```python
from build123d import *

# Parameters (mm, degrees)
SKETCH007_W     = 116.5
SKETCH007_H     = 84
PAD002_DEPTH    = 2
SKETCH008_W     = 112.5
SKETCH008_H     = 80
PAD003_DEPTH    = 2
SKETCH009_W     = 108.5
SKETCH009_H     = 76
POCKET004_DEPTH = 2
FILLET008_R     = 1
FILLET009_R     = 1


with BuildPart() as part:
    # Sketch007 → Pad002 (new body)
    with BuildSketch(Plane(origin=(0, 0, 0), x_dir=(1, 0, 0), z_dir=(0, 0, -1))):
        with Locations((58.25, 42)):
            Rectangle(SKETCH007_W, SKETCH007_H)
    extrude(amount=PAD002_DEPTH)

    # Sketch008 (on Face5 of Pad002) → Pad003 (new body)
    with BuildSketch(Plane.XY):
        with Locations((58.25, -42)):
            Rectangle(SKETCH008_W, SKETCH008_H)
    extrude(amount=PAD003_DEPTH)

    # Sketch009 (on Face11 of Pad003) → Pocket004 (cut)
    with BuildSketch(Plane.XY.offset(2)):
        with Locations((58.25, -42)):
            Rectangle(SKETCH009_W, SKETCH009_H)
    extrude(amount=-POCKET004_DEPTH, mode=Mode.SUBTRACT)

    # Fillet008
    fillet008_edges = [part.edges().sort_by_distance(p)[0] for p in [
        (0, 0, -1),
        (116.5, 0, -1),
        (0, -84, -1),
        (116.5, -84, -1),
        (114.5, -82, 1),
        (2, -82, 1),
        (114.5, -2, 1),
        (2, -2, 1),
    ]]
    fillet(fillet008_edges, radius=FILLET008_R)

    # Fillet009
    fillet009_edges = [part.edges().sort_by_distance(p)[0] for p in [
        (58.25, -2, 2),
    ]]
    fillet(fillet009_edges, radius=FILLET009_R)


solid = part.part
```
The model under review builds one solid part; all positions refer to its coordinate system, in mm. Give positions to 0.01 mm unless a question says otherwise; leave off trailing zeros. Loops run counter-clockwise (first coordinate to the right, second up) from the corner with the lowest first, then second, coordinate; pieces in that order, holes last. Notation, with made-up numbers: (73, -26) - (128, -26) arc R24 ccw to (128, 2) - close; hole circle Ø5 at (-7, -12.5). An arc over 180 degrees is marked (long way). Answer as a JSON object with one key per item and string values.
Q1. Mouldability with a two-part tool opening along Y and no side actions: class faces 1 (the flat face through (57, -41, 0)), 2 (the flat face through (57, -43, -2)) as +Y half, -Y half, draft (parallel to the pull), parting line (faces both ways), or undercut.
Worked out:
{"face 1": "undercut", "face 2": "draft"}
Q2. To check wall thickness, follow line 1 along Y through (x, z) = (92.5, 0.6); line 2 along X through (y, z) = (-41, 0.8); line 3 along Z through (x, y) = (89.5, -61). State the ranges of each line that lie inside material, in increasing order.
Worked out:
{"line 1": "y = -82 to -80, -4 to -2", "line 2": "x = 2 to 4, 112.5 to 114.5", "line 3": "z = -2 to 0"}
Q3. Add section B-B on x = 35.5. State the section outline as (y, z) points.
Worked out:
{"outline": "(-84, -2) - (0, -2) - (0, 0) - (-2, 0) - (-2, 1) arc R1 ccw to (-3, 2) - (-4, 2) - (-4, 0) - (-80, 0) - (-80, 2) - (-81, 2) arc R1 ccw to (-82, 1) - (-82, 0) - (-84, 0) - close"}
Q4. Add section A-A on y = -12. State the section outline as (x, z) points, plus the area to 3 significant figures.
Worked out:
{"outline": "(0, -2) - (116.5, -2) - (116.5, 0) - (114.5, 0) - (114.5, 1) arc R1 ccw to (113.5, 2) - (112.5, 2) - (112.5, 0) - (4, 0) - (4, 2) - (3, 2) arc R1 ccw to (2, 1) - (2, 0) - (0, 0) - close", "area": "241 mm^2"}
Q5. Insertion check: pin 1 (0.5 mm diameter, centred on y = -59.5, z = 0.5, fed in from -X); pin 2 (0.6 mm diameter, centred on x = 39, z = 1.5, fed in from -Y); pin 3 (2 mm diameter, centred on x = 83, z = 1.5, fed in from +Y); pin 4 (2 mm diameter, centred on y = -43, z = 0.5, fed in from +X). Each pin has a flat end and moves straight along its axis. Give the tip position at first contact, or say it passes through.
Worked out:
{"pin 1": "stops at x = 2", "pin 2": "stops at y = -81.98", "pin 3": "stops at y = -2", "pin 4": "stops at x = 116.5"}
